Model file for the job. Use its own axes, mm. A direction names the side the tool comes from. Coordinates: 2 decimals unless noted, no trailing zeros. Write each loop counter-clockwise with the first axis right and the second up, starting at its lowest first coordinate (ties: lowest second). Pieces come first, ordered by that corner, then holes. Notation, with made-up numbers: (45, -29) -> (62, -29) arc R21 ccw to (62, -24) -> close; hole circle Ø7 at (41, 23). An arc over 180 degrees is marked (long way). Write item = value, one per line. Start each with the question number.
from build123d import *

# Parameters (mm, degrees)
SKETCH1_R           = 22.5
BOSS_EXTRUDE1_DEPTH = 10
BOSS_EXTRUDE2_DEPTH = 20
SKETCH3_R           = 16.5
CUT_EXTRUDE2_DEPTH  = 5


with BuildPart() as part:
    # Sketch1 → Boss-Extrude1 (new body)
    with BuildSketch(Plane(origin=(0, 0, 0), x_dir=(1, 0, 0), z_dir=(0, 1, 0))):
        with Locations(Location((0, 0, 0), (0, 0, 270))):
            Circle(SKETCH1_R)
    extrude(amount=BOSS_EXTRUDE1_DEPTH)

    # Sketch2 → Boss-Extrude2 (add)
    with BuildSketch(Plane(origin=(0, 10, 0), x_dir=(1, 0, 0), z_dir=(0, 1, 0))):
        Polygon((-14.828901743, 27.574589589), (13.664688, 27.574589589), (13.664688, 18.076726341), (-5.331038496, 18.076726341), (-5.331038496, 7.90044429), (13.664688, 7.90044429), (13.664688, -1.597418958), (-5.331038496, -1.597418958), (-5.331038496, -15.84421383), (13.664688, -15.84421383), (13.664688, -25.342077078), (-14.828901743, -25.342077078), align=None)
    extrude(amount=BOSS_EXTRUDE2_DEPTH)

    # Sketch3 → Cut-Extrude2 (cut)
    with BuildSketch(Plane.XZ):
        with BuildLine():
            ThreePointArc((-14.551420086, 2.778571429), (0, 11.5), (14.551420086, 2.778571429))
            Line((14.551420086, 2.778571429), (4.83856504, 20.948467447))
            ThreePointArc((4.83856504, 20.948467447), (0, 21.5), (-4.83856504, 20.948467447))
            Line((-4.83856504, 20.948467447), (-14.551420086, 2.778571429))
        make_face()
        with Locations((0, -5)):
            Circle(SKETCH3_R)
    extrude(amount=-CUT_EXTRUDE2_DEPTH, mode=Mode.SUBTRACT)


solid = part.part
(1) Drill centre lines: line 1 along Z through (x, y) = (11, 27.5); line 2 along Y through (x, z) = (13.5, -1.5); line 3 along X through (y, z) = (17.75, -8). Where is each one in solid material? Low to high.
(2) Drop flat-ended pins along their axis: pin 1 Ø3 at (y, z) = (21, 19.5) entering from +X; pin 2 Ø10 at (y, z) = (11, -20) entering from -X; pin 3 Ø10 at (y, z) = (17, -3.5) entering from -X. Give the stop position or say it passes through.
(3) Saw through at B-B (x = 0). Give the cut face in (y, z).
(4) Mould opens along X. For faces 1 (the face through (0, 5, 0)), 2 (the face through (9, 10, 4)), 3 (the face through (-5.331, 20, -13)) say: released by +X, released by -X, zero draft, split by the parting line, or undercut.
(5) Saw through at A-A (y = 12.5). Give the cut face in (x, z).
(6) 3-axis set-ups, long thin cutter, end or side, ignore diameter. For faces 4 (the face through (4, 20, 15.844)), 5 (the face through (0, 10, -25)), 6 (the face through (-18, 10, 0)), 7 (the face through (0.1, 2.5, 21.5)), 8 (the face through (13.665, 20, -3)): which of +Z, -Z, +X, -X, +Y, -Y reach the whole face in a straight line?
(7) Saw through at D-D (x = 10.5). Give the cut face in (y, z), then the cut area to 3 significant figures.
(8) Saw through at C-C (z = 14). Give the cut face in (x, y).
Returned:
q1.line_1 = -27.57 to -18.08, -7.9 to 1.6, 15.84 to 25.34
q1.line_2 = 5 to 30
q1.line_3 = -14.83 to -5.33
q2.pin_1 = 13.66
q2.pin_2 = -16.68
q2.pin_3 = -14.83
q3.outline = (0, -22.5) -> (10, -22.5) -> (10, -27.57) -> (30, -27.57) -> (30, -18.08) -> (10, -18.08) -> (10, -7.9) -> (30, -7.9) -> (30, 1.6) -> (10, 1.6) -> (10, 15.84) -> (30, 15.84) -> (30, 25.34) -> (10, 25.34) -> (10, 22.5) -> (0, 22.5) -> (0, 21.5) -> (5, 21.5) -> (5, -21.5) -> (0, -21.5) -> close
q4.face_1 = undercut
q4.face_2 = zero draft
q4.face_3 = released by +X
q5.outline = (-14.83, -27.57) -> (13.66, -27.57) -> (13.66, -18.08) -> (-5.33, -18.08) -> (-5.33, -7.9) -> (13.66, -7.9) -> (13.66, 1.6) -> (-5.33, 1.6) -> (-5.33, 15.84) -> (13.66, 15.84) -> (13.66, 25.34) -> (-14.83, 25.34) -> close
q6.face_4 = +X, +Y
q6.face_5 = -Z, -Y
q6.face_6 = +Z, -Z, -X, +Y
q6.face_7 = -Y
q6.face_8 = +Z, -Z, +X, +Y
q7.outline = (0, -19.9) -> (10, -19.9) -> (10, -27.57) -> (30, -27.57) -> (30, -18.08) -> (10, -18.08) -> (10, -7.9) -> (30, -7.9) -> (30, 1.6) -> (10, 1.6) -> (10, 15.84) -> (30, 15.84) -> (30, 25.34) -> (10, 25.34) -> (10, 19.9) -> (0, 19.9) -> (0, 10.36) -> (5, 10.36) -> (5, -17.73) -> (0, -17.73) -> close
q7.area = 827 mm2
q8.outline = (-17.61, 0) -> (-8.55, 0) -> (-8.55, 5) -> (8.55, 5) -> (8.55, 0) -> (17.61, 0) -> (17.61, 10) -> (-5.33, 10) -> (-5.33, 30) -> (-14.83, 30) -> (-14.83, 10) -> (-17.61, 10) -> close
